Read the model definition and answer for the solid it produces. Units are mm, in the model's axes. Face numbers are marked on the shaded views. Round coordinates to 2 decimals unless told otherwise and drop trailing zeros. Write each loop counter-clockwise with the first axis right and the second up, starting at its lowest first coordinate (ties: lowest second). Pieces come first, ordered by that corner, then holes. Notation, with made-up numbers: (-32, 55.5) - (-1, 55.5) arc R20 cw to (-1, 69.5) - close; hole circle Ø1 at (21.5, 5). An arc over 180 degrees is marked (long way). Use one line per item in the form item = value. Start each with the question number.
1) The part is cut by section D-D, the plane y = 1.45. Give the vertices of the cut face in (x, z).
2) Consider line 1 along X through (y, z) = (1.3, 0); line 2 along X through (y, z) = (0.5, -1); line 3 along Z through (x, y) = (-0.5, 2.8). Determine where each line is inside the solid, lowest interval first. Write a range as from..to.
3) The part is cut by section B-B, the plane x = -6.35. Give the vertices of the cut face in (y, z).
4) The part is cut by section C-C, the plane z = -14.5. Give the vertices of the cut face in (x, y), plus the area to 3 significant figures.
5) For a pull along X with two mould halves and no side action, classify the marked faces 1, 2, 3 and 4 as released by +X, released by -X, zero draft, split by the parting line, or undercut.
6) The part is cut by section A-A, the plane z = 0. Give the vertices of the cut face in (x, y).
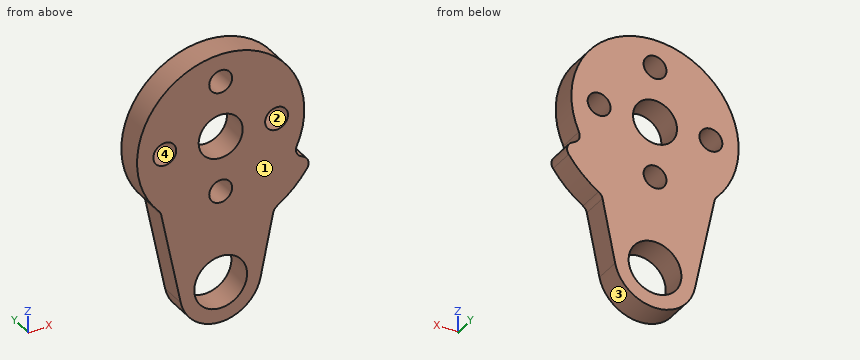
from build123d import *

# Parameters (mm, degrees)
SKETCH1_R           = 3
SKETCH1_R_2         = 2.5
BOSS_EXTRUDE1_DEPTH = 3
SKETCH2_R           = 1.3
CUT_EXTRUDE1_DEPTH  = 3
BOSS_EXTRUDE2_START = -3
BOSS_EXTRUDE2_DEPTH = 3
BOSS_EXTRUDE3_START = -3
BOSS_EXTRUDE3_DEPTH = 3
FILLET1_R           = 1


with BuildPart() as part:
    # Sketch1 → Boss-Extrude1 (new body)
    with BuildSketch(Plane(origin=(0, 0, 0), x_dir=(1, 0, 0), z_dir=(0, 1, 0))):
        with BuildLine():
            Line((-4.531642246, 17.7995776), (-7.838367177, 1.6))
            ThreePointArc((-7.838367177, 1.6), (0, -8), (7.838367177, 1.6))
            Line((7.838367177, 1.6), (4.531642246, 17.7995776))
            ThreePointArc((4.531642246, 17.7995776), (0, 21.499648), (-4.531642246, 17.7995776))
        make_face()
        with Locations(Location((0, 16.87456, 0), (0, 0, 270))):
            Circle(SKETCH1_R, mode=Mode.SUBTRACT)
        with Locations(Location((0, 0, 0), (0, 0, 270))):
            Circle(SKETCH1_R_2, mode=Mode.SUBTRACT)
    extrude(amount=BOSS_EXTRUDE1_DEPTH)

    # Sketch2 → Cut-Extrude1 (cut)
    with BuildSketch(Plane(origin=(0, 3, 0), x_dir=(1, 0, 0), z_dir=(0, 1, 0))):
        with Locations(Location((0, 6.35, 0), (0, 0, 270))):
            Circle(SKETCH2_R)
        with Locations(Location((6.35, 0, 0), (0, 0, 270))):
            Circle(SKETCH2_R)
        with Locations(Location((0, -6.35, 0), (0, 0, 270))):
            Circle(SKETCH2_R)
        with Locations(Location((-6.35, 0, 0), (0, 0, 270))):
            Circle(SKETCH2_R)
    extrude(amount=-CUT_EXTRUDE1_DEPTH, mode=Mode.SUBTRACT)

    # Sketch3 → Boss-Extrude2 (add)
    with BuildSketch(Plane(origin=(0, 3, 0), x_dir=(1, 0, 0), z_dir=(0, 1, 0)).offset(BOSS_EXTRUDE2_START)):
        with BuildLine():
            Line((-7.838367177, 1.6), (-6.8136721, 6.619960159))
            ThreePointArc((-6.8136721, 6.619960159), (0, -9.5), (6.8136721, 6.619960159))
            Line((6.8136721, 6.619960159), (7.838367177, 1.6))
            ThreePointArc((7.838367177, 1.6), (0, -8), (-7.838367177, 1.6))
        make_face()
    extrude(amount=BOSS_EXTRUDE2_DEPTH)

    # Sketch4 → Boss-Extrude3 (add)
    with BuildSketch(Plane(origin=(0, 3, 0), x_dir=(1, 0, 0), z_dir=(0, 1, 0)).offset(BOSS_EXTRUDE3_START)):
        with BuildLine():
            Line((8.227241336, 4.75), (10.392304845, 6))
            ThreePointArc((10.392304845, 6), (6, 10.392304845), (0, 12))
            Line((0, 12), (0, 9.5))
            ThreePointArc((0, 9.5), (4.75, 8.227241336), (8.227241336, 4.75))
        make_face()
    extrude(amount=BOSS_EXTRUDE3_DEPTH)

    # Fillet1
    fillet1_edges = [part.edges().sort_by_distance(p)[0] for p in [
        (-6.8136721, 1.5, -6.619960159),
        (6.049512795, 1.5, -10.36356092),
        (8.227241336, 1.5, -4.75),
        (10.392304845, 1.5, -6),
    ]]
    fillet(fillet1_edges, radius=FILLET1_R)


solid = part.part
Geometry results:
q1.outline = (-7, -6.42) arc R1 cw to (-6.76, -6.9) - (-4.53, -17.8) arc R4.63 ccw to (4.53, -17.8) - (5.96, -10.79) arc R1 cw to (6.41, -10.15) arc R12 ccw to (9.8, -6.92) arc R1 ccw to (9.49, -5.48) - (9.05, -5.23) arc R1 cw to (8.64, -3.94) arc R9.5 ccw (long way) to start; hole circle Ø2.6 at (-6.35, 0); hole circle Ø6 at (0, -16.87); hole circle Ø5 at (0, 0); hole circle Ø2.6 at (0, -6.35); hole circle Ø2.6 at (0, 6.35); hole circle Ø2.6 at (6.35, 0)
q2.line_1 = -9.5..-7.65, -5.05..-2.5, 2.5..5.05, 7.65..9.5
q2.line_2 = -9.45..-7.18, -5.52..-2.29, 2.29..5.52, 7.18..9.45
q2.line_3 = -21.47..-19.83, -13.92..-7.55, -5.15..-2.45, 2.45..5.15, 7.55..9.49
q3.outline = (0, -8.89) - (3, -8.89) - (3, -1.3) - (0, -1.3) - close; (0, 1.3) - (3, 1.3) - (3, 7.07) - (0, 7.07) - close
q4.outline = (-5.21, 0) - (-1.83, 0) - (-1.83, 3) - (-5.21, 3) - close; (1.83, 0) - (5.21, 0) - (5.21, 3) - (1.83, 3) - close
q4.area = 20.2 mm2
q5.face_1 = zero draft
q5.face_2 = undercut
q5.face_3 = split by the parting line
q5.face_4 = undercut
q6.outline = (-9.5, 0) - (-7.65, 0) - (-7.65, 3) - (-9.5, 3) - close; (-5.05, 0) - (-2.5, 0) - (-2.5, 3) - (-5.05, 3) - close; (2.5, 0) - (5.05, 0) - (5.05, 3) - (2.5, 3) - close; (7.65, 0) - (9.5, 0) - (9.5, 3) - (7.65, 3) - close
